```python
from build123d import *

# Parameters (mm, degrees)
CYLINDER682_R               = 8
CYLINDER682_DEPTH           = 6
CYLINDER669_R               = 1.5
CYLINDER669_DEPTH           = 50
CYLINDER669_PLACEMENT_ANGLE = 45
CYLINDER672_R               = 1.5
CYLINDER672_DEPTH           = 50
CYLINDER672_PLACEMENT_ANGLE = 45
CYLINDER680_R               = 1.5
CYLINDER680_DEPTH           = 50
CYLINDER680_PLACEMENT_ANGLE = 45
CYLINDER673_R               = 1.5
CYLINDER673_DEPTH           = 50
CYLINDER673_PLACEMENT_ANGLE = 45
BOX249_W                    = 68
BOX249_H                    = 36
BOX249_DEPTH                = 4


with BuildPart() as obj1:
    # Cylinder682 → Cylinder682 (new body)
    with BuildSketch(Plane(origin=(0, 83, 25), x_dir=(1, 0, 0), z_dir=(0, 0, 1))):
        Circle(CYLINDER682_R)
    extrude(amount=CYLINDER682_DEPTH)


with BuildPart() as obj2:
    # Cylinder669 → Cylinder669 (new body)
    with BuildSketch(Plane.XY):
        Circle(CYLINDER669_R)
    extrude(amount=CYLINDER669_DEPTH)


with BuildPart() as obj2_1:
    # Cylinder669 placement: moved
    add(obj2.part.moved(Location((-31, 92, 0))).rotate(Axis((-31, 92, 0), (0, 0, 1)), CYLINDER669_PLACEMENT_ANGLE))


with BuildPart() as obj3:
    # Cylinder672 → Cylinder672 (new body)
    with BuildSketch(Plane.XY):
        Circle(CYLINDER672_R)
    extrude(amount=CYLINDER672_DEPTH)


with BuildPart() as obj3_1:
    # Cylinder672 placement: moved
    add(obj3.part.moved(Location((31, 110, 0))).rotate(Axis((31, 110, 0), (0, 0, 1)), CYLINDER672_PLACEMENT_ANGLE))


with BuildPart() as obj4:
    # Cylinder680 → Cylinder680 (new body)
    with BuildSketch(Plane.XY):
        Circle(CYLINDER680_R)
    extrude(amount=CYLINDER680_DEPTH)


with BuildPart() as obj4_1:
    # Cylinder680 placement: moved
    add(obj4.part.moved(Location((31, 92, 0))).rotate(Axis((31, 92, 0), (0, 0, 1)), CYLINDER680_PLACEMENT_ANGLE))


with BuildPart() as compound397:
    # Cylinder673 → Cylinder673 (new body)
    with BuildSketch(Plane.XY):
        Circle(CYLINDER673_R)
    extrude(amount=CYLINDER673_DEPTH)


with BuildPart() as compound397_1:
    # Cylinder673 placement: moved
    add(compound397.part.moved(Location((-31, 110, 0))).rotate(Axis((-31, 110, 0), (0, 0, 1)), CYLINDER673_PLACEMENT_ANGLE))

    # Compound397: union obj2, obj3, obj4
    add(obj2_1.part)
    add(obj3_1.part)
    add(obj4_1.part)


with BuildPart() as cut266:
    # Box249 → Box249 (new body)
    with BuildSketch(Plane(origin=(-34, 86, 27), x_dir=(1, 0, 0), z_dir=(0, 0, 1))):
        with Locations((34, 18)):
            Rectangle(BOX249_W, BOX249_H)
    extrude(amount=BOX249_DEPTH)

    # Cut276: cut Compound397
    add(compound397_1.part, mode=Mode.SUBTRACT)

    # Cut266: cut obj1
    add(obj1.part, mode=Mode.SUBTRACT)


solid = cut266.part
```
Could you check a few things on this model? Use its own coordinates, in mm. Coordinates: 2 decimals unless noted, no trailing zeros. Order: outer loops, then holes, each group sorted by start corner. A loop starts at its lowest first (then second) coordinate and runs counter-clockwise, first axis right, second up. Notation, with made-up numbers: M 7,18 L 35,18 A28 ccw 35,52 Z; hole C 47,72 d11. An arc over 180 degrees is marked long. Use one line per item in the form item = value. Start each with the question number.
1. Please list where these lines run through material, in increasing order: line 1 (X direction, y = 110, z = 28.85); line 2 (Y direction, x = 31, z = 29.15); line 3 (Y direction, x = -3, z = 27.4).
2. For pin 1 (2.5 mm diameter, centred on x = -31, y = 92, fed in from +Z), with a flat end and sliding along its axis, tell me the tip position at first contact or that it passes through.
3. We'd pull the mould along Y, two halves only. Please class faces 1 (the flat face through (21, 86, 29)), 2 (the flat face through (0, 104, 31)), 3 (the cylindrical face through (30.804, 108.513, 28.972)): +Y half, -Y half, draft (parallel to the pull), parting line (faces both ways), or undercut.
4. Suppose I cut it at B-B on y = 92. Write out the boundary of the cut face in (x, z), then the cut area to 3 significant figures.
5. Suppose I cut it at C-C on z = 28.25. Write out the boundary of the cut face in (x, y).
6. Suppose I cut it at A-A on x = 31. Write out the boundary of the cut face in (y, z).
Geometry says:
q1.line_1 = -34 to -32.5, -29.5 to 29.5, 32.5 to 34
q1.line_2 = 86 to 90.5, 93.5 to 108.5, 111.5 to 122
q1.line_3 = 90.42 to 122
q2.pin_1 = through
q3.face_1 = -Y half
q3.face_2 = draft
q3.face_3 = undercut
q4.outline = M -34,27 L -32.5,27 L -32.5,31 L -34,31 Z; M -29.5,27 L 29.5,27 L 29.5,31 L -29.5,31 Z; M 32.5,27 L 34,27 L 34,31 L 32.5,31 Z
q4.area = 248 mm^2
q5.outline = M -34,86 L -7.42,86 A8 cw 7.42,86 L 34,86 L 34,122 L -34,122 Z; hole C -31,92 d3; hole C -31,110 d3; hole C 31,92 d3; hole C 31,110 d3
q6.outline = M 86,27 L 90.5,27 L 90.5,31 L 86,31 Z; M 93.5,27 L 108.5,27 L 108.5,31 L 93.5,31 Z; M 111.5,27 L 122,27 L 122,31 L 111.5,31 Z
